Study the drawing (mm; zero at the part's minimum x, y, z) and answer. Give positions to 0.01 mm unless a question says otherwise; leave off trailing zeros. Write each loop counter-clockwise with the first axis right and the second up, starting at its lowest first coordinate (ties: lowest second). Pieces come first, ordered by that corner, then holes. Notation, with made-up numbers: (12, -22) -> (21, -22) arc R21 cw to (21, -11) -> close; hole circle Ø4 at (77, 23.5). An arc over 180 degrees is marked (long way). Put each result on its own line as item: value. Start each with the question number.
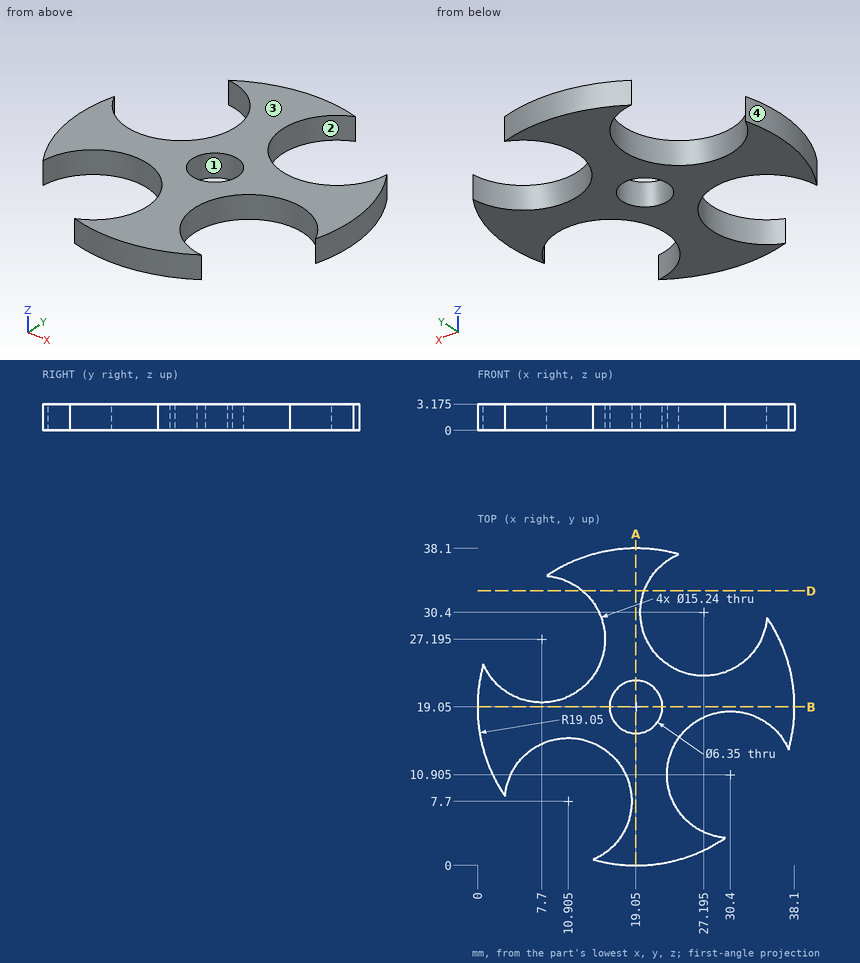
1) A cutting plane is placed at D-D on y = 33. Give the vertices of the cut face in (x, z) (1 decimal).
2) A cutting plane is placed at A-A on x = 19.05. Give the vertices of the cut face in (y, z) (1 decimal).
3) For a pull along Y with two mould halves and no side action, classify the marked faces 1, 2, 3 and 4 as pulls with the +Y half, pulls with the -Y half, needs draft (parallel to the pull), parting line crosses it, or undercut.
4) Each of these flat-tipped pins is pushed along its axis until it touches: pin 1 Ø20 at (x, y) = (30.4, 10.91) entering from +Z (3 decimals); pin 2 Ø1.5 at (y, z) = (33, 2.5) entering from +X; pin 3 Ø1 at (x, z) = (24, 1) entering from -Y. Where does it stop, or does it pass through?
5) Straight lines are drawn through the part: line 1 (X direction, y = 17, z = 2.4) (1 decimal); line 2 (X direction, y = 19, z = 0.5) (1 decimal). For each, find the intervals that lie inside material, in ascending order. Write a range as [from, to].
Results found:
1. outline: (12.6, 0) -> (20, 0) -> (20, 3.2) -> (12.6, 3.2) -> close
2. outline: (0, 0) -> (15.9, 0) -> (15.9, 3.2) -> (0, 3.2) -> close; (22.2, 0) -> (38.1, 0) -> (38.1, 3.2) -> (22.2, 3.2) -> close
3. face 1: undercut
3. face 2: undercut
3. face 3: needs draft
3. face 4: parting line crosses it
4. pin 1: stops at z = 3.175
4. pin 2: stops at x = 20.35
4. pin 3: stops at y = 0.53
5. line 1: x = [0.1, 16.6], [21.5, 25.8], [35, 38]
5. line 2: x = [0, 15.9], [22.2, 38.1]
